```python
from build123d import *

# Parameters (mm, degrees)
F1_DEPTH = 3.175


with BuildPart() as f1:
    # F0 (on Front) → F1 (new body, symmetric)
    with BuildSketch(Plane.XZ):
        with BuildLine():
            Line((4.7625, 107.95), (-4.7625, 107.95))
            ThreePointArc((-4.7625, 107.95), (-9.252628, 106.090128), (-11.1125, 101.6))
            Line((-11.1125, 101.6), (-11.1125, 47.625))
            ThreePointArc((-11.1125, 47.625), (-12.042436, 45.379936), (-14.2875, 44.45))
            ThreePointArc((-14.2875, 44.45), (-21.022692, 41.660192), (-23.8125, 34.925))
            Line((-23.8125, 34.925), (-23.8125, -44.45))
            Line((-23.8125, -44.45), (-3.175, -44.45))
            Line((-3.175, -44.45), (-3.175, 50.8))
            Line((-3.175, 50.8), (3.175, 50.8))
            Line((3.175, 50.8), (3.175, -44.45))
            Line((3.175, -44.45), (23.8125, -44.45))
            Line((23.8125, -44.45), (23.8125, 34.925))
            ThreePointArc((23.8125, 34.925), (21.022692, 41.660192), (14.2875, 44.45))
            ThreePointArc((14.2875, 44.45), (12.042436, 45.379936), (11.1125, 47.625))
            Line((11.1125, 47.625), (11.1125, 101.6))
            ThreePointArc((11.1125, 101.6), (9.252628, 106.090128), (4.7625, 107.95))
        make_face()
    extrude(amount=F1_DEPTH, both=True)


solid = f1.part
```
CAD build for the part. Positions are in the model's coordinates, mm. A direction names the side the tool comes from. Coordinates: 2 decimals unless noted, no trailing zeros. Loops run counter-clockwise (first coordinate to the right, second up) from the corner with the lowest first, then second, coordinate; pieces in that order, holes last. Notation, with made-up numbers: (21.5, 4.25) - (79.5, 4.25) arc R5 cw to (79.5, 12.25) - close; hole circle Ø7 at (84.5, 20.5). An arc over 180 degrees is marked (long way). Use CSV: the item, a comma, the result in double quotes. Start each with the question number.
Q1. 3-axis set-ups, long thin cutter, end or side, ignore diameter. For faces 1 (the flat face through (11.112, 0, 74)), 2 (the flat face through (13, 0, -44.45)), 3 (the flat face through (-3.175, 0, 3)): which of +Z, -Z, +X, -X, +Y, -Y reach the whole face in a straight line?
Q2. Cut at C-C, the plane z = 37.5. List the corners of the cut face in (x, y) (3 decimals).
Q3. Drop flat-ended pins along their axis: P1, Ø2, axis at y = 2, z = 35.5, coming from the -X side; P2, Ø3, axis at y = 1, z = 66, coming from the +X side; P3, Ø2, axis at x = -14.5, y = 2, coming from the +Z side. Give the stop position or say it passes through.
Q4. Two-plate mould, pull along X, no slides. Class faces 4 (the flat face through (5, 3.175, 16)), 5 (the flat face through (0, 0, 50.8)), 6 (the flat face through (-11.112, 0, 75)): +X half, -X half, draft (parallel to the pull), parting line (faces both ways), or undercut.
Q5. Cut at A-A, the plane z = 2. List the corners of the cut face in (x, y) (1 decimal).
Q6. Cut at D-D, the plane x = -17.5. List the corners of the cut face in (y, z) (3 decimals), then the cut area to 3 significant figures.
Q7. Probe probe 1 along X at (y, z) = (-0.25, -9) (1 decimal); probe 2 along X at (y, z) = (-2.5, 52.5); probe 3 along Z at (x, y) = (2, 2.75). List the from-to ranges inside material, lowest first. Write a range as from..to.
Here are the results:
1,face 1,"+Z, +X, +Y, -Y"
1,face 2,"-Z, +X, -X, +Y, -Y"
1,face 3,"-Z, +Y, -Y"
2,outline,"(-23.458, -3.175) - (-3.175, -3.175) - (-3.175, 3.175) - (-23.458, 3.175) - close; (3.175, -3.175) - (23.458, -3.175) - (23.458, 3.175) - (3.175, 3.175) - close"
3,P1,"x = -23.81"
3,P2,"x = 11.11"
3,P3,"z = 44.55"
4,face 4,"draft"
4,face 5,"undercut"
4,face 6,"-X half"
5,outline,"(-23.8, -3.2) - (-3.2, -3.2) - (-3.2, 3.2) - (-23.8, 3.2) - close; (3.2, -3.2) - (23.8, -3.2) - (23.8, 3.2) - (3.2, 3.2) - close"
6,outline,"(-3.175, -44.45) - (3.175, -44.45) - (3.175, 43.892) - (-3.175, 43.892) - close"
6,area,"561 mm2"
7,probe 1,"-23.8..-3.2, 3.2..23.8"
7,probe 2,"-11.11..11.11"
7,probe 3,"50.8..107.95"
